Design review of the part built by this model. Coordinates are the model's own, in mm. A direction names the side the tool comes from. Give positions to 0.01 mm unless a question says otherwise; leave off trailing zeros. Loops run counter-clockwise (first coordinate to the right, second up) from the corner with the lowest first, then second, coordinate; pieces in that order, holes last. Notation, with made-up numbers: (-38, 38) -> (-16, 38) arc R9 cw to (-16, 54) -> close; hole circle Ø7 at (42.25, 87). An arc over 180 degrees is marked (long way). Answer in a Markdown table with one row per item. Add a question column.
(1) Draft analysis for pull direction X (two halves, no side actions). For faces 1 (the flat face through (-1, 0, -10)), 2 (the flat face through (-2.7, -6.5, -7.5)), 3 (the flat face through (28.5, -3, 0)), state which applies: +X half, -X half, draft (parallel to the pull), parting line (faces both ways), or undercut.
(2) Consider section C-C on z = 0. Write out the cut boundary in (x, y), then the cut area to 3 significant figures.
(3) Consider section A-A on x = -2. Write out the cut boundary in (y, z), then the cut area to 3 significant figures.
(4) For faces 4 (the flat face through (27.5, -4, 0)), 5 (the cylindrical face through (22.43, -6.49, -0.65)), 6 (the cylindrical face through (17.5, -6.49, -0.16)), 7 (the flat face through (-27.5, -0.5, 0.2)), 8 (the cylindrical face through (27.98, -0.5, -0.21)), list the 3-axis set-ups (+Z, -Z, +X, -X, +Y, -Y) from which the entire face can be reached by the end or side of a thin tool; tool diameter is ignored.
(5) Consider section B-B on z = 6. Write out the cut boundary in (x, y), then the cut area to 3 significant figures.
(6) Consider section D-D on x = 24. Write out the cut boundary in (y, z), then the cut area to 3 significant figures.
(7) For pin 1 (4 mm diameter, centred on x = -10.5, z = 4.5, fed in from +Y), flat-tipped, find the tip position at first contact; note if it passes through.
(8) For line 1 (Z direction, x = 24, y = -6.8); line 2 (Y direction, x = -23, z = -10.75); line 3 (Z direction, x = 0, y = -6.25), list the stretches that pass through material, from the lowest coordinate up.
from build123d import *

# Parameters (mm, degrees)
ESQUISSE2_W                           = 55
ESQUISSE2_H                           = 30
T_LE_DE_BASE_PLI_E1_DEPTH             = 1
T_LE_PLI_E_SUR_AR_TE1_STRIP_W         = 5.4732
T_LE_PLI_E_SUR_AR_TE1_STRIP_H         = 1
T_LE_PLI_E_SUR_AR_TE1_STRIP_CUT_DEPTH = 30
T_LE_PLI_E_SUR_AR_TE1_DEPTH           = 30
T_LE_PLI_E_SUR_AR_TE2_STRIP_W         = 5.4732
T_LE_PLI_E_SUR_AR_TE2_STRIP_H         = 1
T_LE_PLI_E_SUR_AR_TE2_STRIP_CUT_DEPTH = 30
T_LE_PLI_E_SUR_AR_TE2_DEPTH           = 30
ENL_V_MAT_EXTRU_1_DEPTH               = 33.958306995
ESQUISSE29_R                          = 1.7
ENL_V_MAT_EXTRU_3_DEPTH               = 33.760494502


# Sheet-metal steps are written as plain solids
with BuildPart() as part:
    # Esquisse2 → Tôle de base pliée1 (new body)
    with BuildSketch(Plane(origin=(0, 0, 0), x_dir=(1, 0, 0), z_dir=(0, 1, 0))):
        Rectangle(ESQUISSE2_W, ESQUISSE2_H)
    extrude(amount=-T_LE_DE_BASE_PLI_E1_DEPTH)

    # Tôle pliée sur arête1 strip (across the edge) → Tôle pliée sur arête1 strip cut (cut)
    with BuildSketch(Plane(origin=(27.5, -1, -15), x_dir=(-1, 0, 0), z_dir=(0, 0, 1))):
        with Locations((-2, -0.5)):
            Rectangle(T_LE_PLI_E_SUR_AR_TE1_STRIP_W, T_LE_PLI_E_SUR_AR_TE1_STRIP_H)
    extrude(amount=T_LE_PLI_E_SUR_AR_TE1_STRIP_CUT_DEPTH, mode=Mode.SUBTRACT)

    # Tôle pliée sur arête1 section (across the edge) → Tôle pliée sur arête1 (add)
    with BuildSketch(Plane(origin=(27.5, -1, -15), x_dir=(-1, 0, 0), z_dir=(0, 0, 1))):
        with BuildLine():
            Line((-1, 0.7366), (-1, 5))
            Line((-1, 5), (0, 5))
            Line((0, 5), (0, 0.7366))
            ThreePointArc((0, 0.7366), (0.215745145, 0.215745145), (0.7366, 0))
            Line((0.7366, 0), (0.7366, -1))
            ThreePointArc((0.7366, -1), (-0.491361636, -0.491361636), (-1, 0.7366))
        make_face()
    extrude(amount=T_LE_PLI_E_SUR_AR_TE1_DEPTH)

    # Tôle pliée sur arête2 strip (across the edge) → Tôle pliée sur arête2 strip cut (cut)
    with BuildSketch(Plane(origin=(27.5, -6, -15), x_dir=(0, 1, 0), z_dir=(0, 0, 1))):
        with Locations((-2, -0.5)):
            Rectangle(T_LE_PLI_E_SUR_AR_TE2_STRIP_W, T_LE_PLI_E_SUR_AR_TE2_STRIP_H)
    extrude(amount=T_LE_PLI_E_SUR_AR_TE2_STRIP_CUT_DEPTH, mode=Mode.SUBTRACT)

    # Tôle pliée sur arête2 section (across the edge) → Tôle pliée sur arête2 (add)
    with BuildSketch(Plane(origin=(27.5, -6, -15), x_dir=(0, 1, 0), z_dir=(0, 0, 1))):
        with BuildLine():
            Line((-1, 0.7366), (-1, 55))
            Line((-1, 55), (0, 55))
            Line((0, 55), (0, 0.7366))
            ThreePointArc((0, 0.7366), (0.215745145, 0.215745145), (0.7366, 0))
            Line((0.7366, 0), (0.7366, -1))
            ThreePointArc((0.7366, -1), (-0.491361636, -0.491361636), (-1, 0.7366))
        make_face()
    extrude(amount=T_LE_PLI_E_SUR_AR_TE2_DEPTH)

    # Esquisse26 → Enlèv. mat.-Extru.1 (cut, through all)
    with BuildSketch(Plane(origin=(0, 0, 0), x_dir=(1, 0, 0), z_dir=(0, 1, 0))):
        with BuildLine():
            Line((-15, 7.5), (10, 7.5))
            ThreePointArc((10, 7.5), (17.5, 0), (10, -7.5))
            Line((10, -7.5), (-15, -7.5))
            ThreePointArc((-15, -7.5), (-22.5, 0), (-15, 7.5))
        make_face()
    extrude(amount=-ENL_V_MAT_EXTRU_1_DEPTH, mode=Mode.SUBTRACT)

    # Esquisse29 → Enlèv. mat.-Extru.3 (cut, through all)
    with BuildSketch(Plane(origin=(0, -6, 0), x_dir=(1, 0, 0), z_dir=(0, 1, 0))):
        with Locations(Location((24, 0, 0), (0, 0, 180))):
            Circle(ESQUISSE29_R)
    extrude(amount=-ENL_V_MAT_EXTRU_3_DEPTH, mode=Mode.SUBTRACT)


solid = part.part
Values follow:
| question | item | result |
|---|---|---|
| 1 | face 1 | draft |
| 1 | face 2 | undercut |
| 1 | face 3 | +X half |
| 2 | outline | (-27.5, -7) -> (-22.5, -7) -> (-22.5, -6) -> (-27.5, -6) -> close; (-27.5, -1) -> (-22.5, -1) -> (-22.5, 0) -> (-27.5, 0) -> close; (17.5, -7) -> (22.3, -7) -> (22.3, -6) -> (17.5, -6) -> close; (17.5, -1) -> (26.76, -1) arc R0.74 cw to (27.5, -1.74) -> (27.5, -5.26) arc R0.74 cw to (26.76, -6) -> (25.7, -6) -> (25.7, -7) -> (26.76, -7) arc R1.74 ccw to (28.5, -5.26) -> (28.5, -1.74) arc R1.74 ccw to (26.76, 0) -> (17.5, 0) -> close |
| 2 | area | 32.5 mm2 |
| 3 | outline | (-7, -15) -> (-6, -15) -> (-6, -7.5) -> (-7, -7.5) -> close; (-7, 7.5) -> (-6, 7.5) -> (-6, 15) -> (-7, 15) -> close; (-1, -15) -> (0, -15) -> (0, -7.5) -> (-1, -7.5) -> close; (-1, 7.5) -> (0, 7.5) -> (0, 15) -> (-1, 15) -> close |
| 3 | area | 30.0 mm2 |
| 4 | face 4 | +Z, -Z, -X |
| 4 | face 5 | -Y |
| 4 | face 6 | +Y, -Y |
| 4 | face 7 | +Z, -Z, -X, +Y, -Y |
| 4 | face 8 | +Z, -Z, +X, +Y |
| 5 | outline | (-27.5, -7) -> (-19.5, -7) -> (-19.5, -6) -> (-27.5, -6) -> close; (-27.5, -1) -> (-19.5, -1) -> (-19.5, 0) -> (-27.5, 0) -> close; (14.5, -7) -> (26.76, -7) arc R1.74 ccw to (28.5, -5.26) -> (28.5, -1.74) arc R1.74 ccw to (26.76, 0) -> (14.5, 0) -> (14.5, -1) -> (26.76, -1) arc R0.74 cw to (27.5, -1.74) -> (27.5, -5.26) arc R0.74 cw to (26.76, -6) -> (14.5, -6) -> close |
| 5 | area | 47.9 mm2 |
| 6 | outline | (-7, -15) -> (-6, -15) -> (-6, -1.7) -> (-7, -1.7) -> close; (-7, 1.7) -> (-6, 1.7) -> (-6, 15) -> (-7, 15) -> close; (-1, -15) -> (0, -15) -> (0, 15) -> (-1, 15) -> close |
| 6 | area | 56.6 mm2 |
| 7 | pin 1 | through |
| 8 | line 1 | -15 to -1.7, 1.7 to 15 |
| 8 | line 2 | -7 to -6, -1 to 0 |
| 8 | line 3 | -15 to -7.5, 7.5 to 15 |
